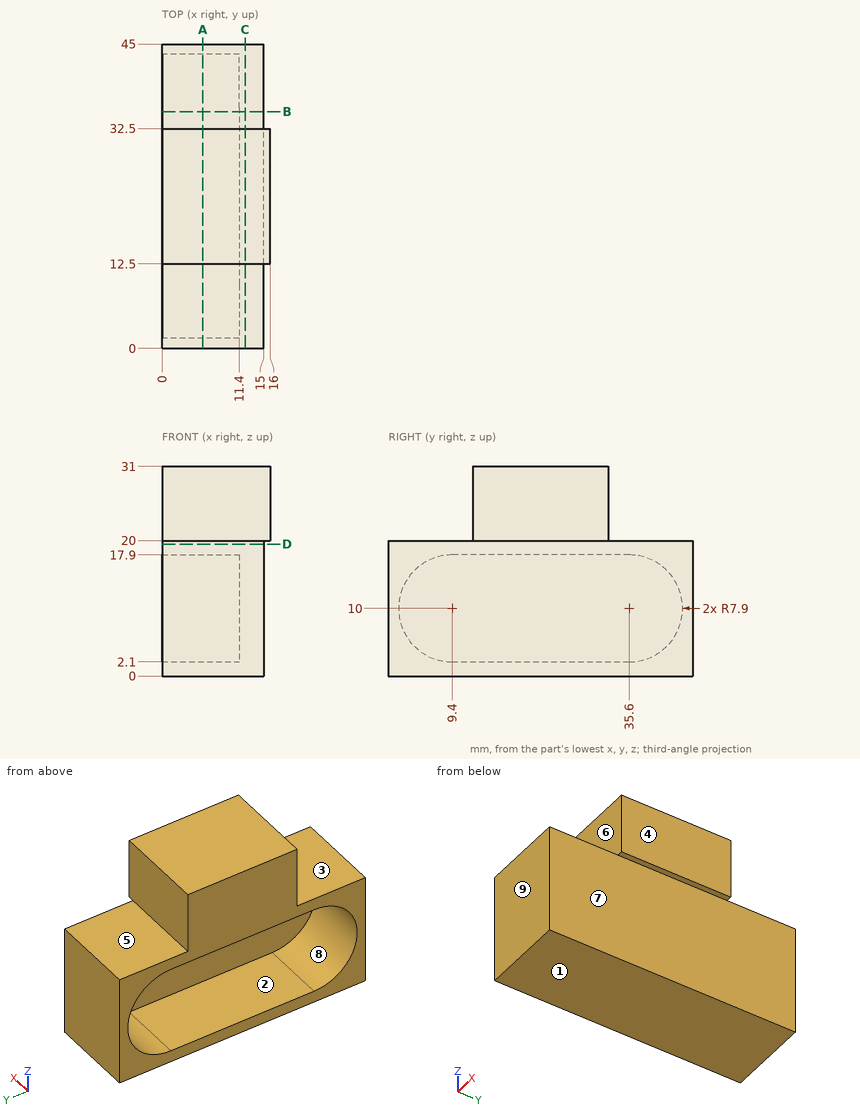
Source: three-view drawing plus pictorial views. Frame: mm from the lowest corner of the part. A direction names the side the tool comes from. Give positions to 0.01 mm unless a question says otherwise; leave off trailing zeros. Write each loop counter-clockwise with the first axis right and the second up, starting at its lowest first coordinate (ties: lowest second). Pieces come first, ordered by that corner, then holes.
(1) Access query for the marked faces 5, 6, 7, 8 and 9. Directions: +Z, -Z, +X, -X, +Y, -Y. A direction counts if a zero-diameter tool reaches every point of the face in a straight line with its end or side. Return the directions, or none.
(2) First-contact query: P1, Ø9, axis at x = 10.5, z = 26, coming from the +Y side; P2, Ø6, axis at x = 7.5, y = 39.5, coming from the +Z side; P3, Ø5.5, axis at x = 7, z = 25, coming from the -Y side. Flat tips, straight axial feed; report the tip coordinate or a pass-through.
(3) Mould query, pull axis Z, two halves, no side actions, for the marked faces 1, 2, 3 and 4. Classes: released by +Z, released by -Z, zero draft, split by the parting line, or undercut.
(4) Ray query, line 1 (Z direction, x = 11, y = 16); line 2 (Z direction, x = 7, y = 35); line 3 (X direction, y = 15.5, z = 8). Return the intervals inside material, ascending.
(5) Cut plane D-D, the plane z = 19.5. Return loops of the section in (x, y), then the cut area to 3 significant figures.
(6) Cut plane A-A, the plane x = 6. Return loops of the section in (y, z).
(7) Cut plane C-C, the plane x = 12.25. Return loops of the section in (y, z), then the cut area to 3 significant figures.
(8) Cut plane B-B, the plane y = 35. Return loops of the section in (x, z), then the cut area to 3 significant figures.
Values follow:
1. face 5: +Z, +X, -X, +Y
1. face 6: +Z, +X, -X, -Y
1. face 7: -Z, +X, +Y, -Y
1. face 8: -X
1. face 9: +Z, -Z, +X, -X, -Y
2. P1: stops at y = 32.5
2. P2: stops at z = 20
2. P3: stops at y = 12.5
3. face 1: released by -Z
3. face 2: undercut
3. face 3: released by +Z
3. face 4: zero draft
4. line 1: z = 0 to 2.1, 17.9 to 31
4. line 2: z = 0 to 2.1, 17.9 to 20
4. line 3: x = 11.4 to 15
5. outline: (0, 0) - (15, 0) - (15, 45) - (0, 45) - close
5. area: 675 mm2
6. outline: (0, 0) - (45, 0) - (45, 20) - (32.5, 20) - (32.5, 31) - (12.5, 31) - (12.5, 20) - (0, 20) - close; hole (9.4, 2.1) - (35.6, 2.1) arc R7.9 ccw to (35.6, 17.9) - (9.4, 17.9) arc R7.9 ccw to start
7. outline: (0, 0) - (45, 0) - (45, 20) - (32.5, 20) - (32.5, 31) - (12.5, 31) - (12.5, 20) - (0, 20) - close
7. area: 1,120 mm2
8. outline: (0, 0) - (15, 0) - (15, 20) - (0, 20) - (0, 17.9) - (11.4, 17.9) - (11.4, 2.1) - (0, 2.1) - close
8. area: 120 mm2
